```python
from build123d import *

# Parameters (mm, degrees)
F1_DEPTH = 9.525
F2_R     = 2
F3_DEPTH = 1.6002
F5_DEPTH = 1.6002
F6_R     = 2.0447
F6_R_2   = 2.05
F7_DEPTH = 1.6002


# Not quite as in the source:
# - a feature names something its author has since deleted; it is built from what else it names


with BuildPart() as f1:
    # F0 (on Front) → F1 (new body, symmetric)
    with BuildSketch(Plane.XZ):
        Polygon((1.6002, 19.05), (0, 19.05), (0, 0), (20.6502, 0), (20.6502, 1.6002), (1.6002, 1.6002), align=None)
    extrude(amount=F1_DEPTH, both=True)

    # F2 (on face) → F3 (cut, through all)
    with BuildSketch(Plane(origin=(0, 0, 0), x_dir=(0, -1, 0), z_dir=(-1, 0, 0))):
        with Locations((0, 11.43)):
            Circle(F2_R)
    extrude(amount=-F3_DEPTH, mode=Mode.SUBTRACT)

    # F4 (on face) → F5 (cut, through all)
    with BuildSketch(Plane(origin=(0, 0, 0), x_dir=(0, -1, 0), z_dir=(-1, 0, 0))):
        with BuildLine():
            Line((-9.525, 19.05), (-9.525, 1.6002))
            Line((-9.525, 1.6002), (-4.6136292969, 13.3572842838))
            ThreePointArc((-4.6136292969, 13.3572842838), (-2.7716041006, 15.5915154343), (0, 16.43))
            ThreePointArc((0, 16.43), (2.7716041006, 15.5915154343), (4.6136292969, 13.3572842838))
            Line((4.6136292969, 13.3572842838), (9.525, 1.6002))
            Line((9.525, 1.6002), (9.525, 19.05))
            Line((9.525, 19.05), (-9.525, 19.05))
        make_face()
    extrude(amount=-F5_DEPTH, mode=Mode.SUBTRACT)

    # F6 (on face) → F7 (cut, through all)
    with BuildSketch(Plane.XY.offset(1.6002)):
        with Locations((13.0302, 5.08)):
            Circle(F6_R)
        with Locations((9.2202, -4.445)):
            Circle(F6_R_2)
    extrude(amount=-F7_DEPTH, mode=Mode.SUBTRACT)


solid = f1.part
```
Check sheet for the modelled part. Datum: model origin and axes. Units: mm. A direction names the side the tool comes from. Coordinates: 2 decimals unless noted, no trailing zeros. Order: outer loops, then holes, each group sorted by start corner. A loop starts at its lowest first (then second) coordinate and runs counter-clockwise, first axis right, second up. Notation, with made-up numbers: (-35, 24) -> (-13, 24) arc R4 ccw to (-13, 30) -> close; hole circle Ø11 at (7.5, -14.5). An arc over 180 degrees is marked (long way). Write each question's results on one line, items separated by ' | '. Start each with the question number.
1) Section check C-C (x = 13). Enter the section's corners in (y, z) (3 decimals).
2) Draft check along X on faces 1 (the face through (0.789, -7.035, 7.561)), 2 (the face through (10.987, 5.17, 0.811)), 3 (the face through (0, 0, 7)). Enter one of: pulls with the +X half, pulls with the -X half, needs draft (parallel to the pull), parting line crosses it, or undercut.
3) Set-up check for faces 4 (the face through (0.789, 0.26, 13.413)), 5 (the face through (11, 0, 1.6)): record each of +Z, -Z, +X, -X, +Y, -Y from which the full face is reachable in a straight line by a thin tool's end or side.
4) Section check D-D (x = 16). Enter the section's corners in (y, z) (3 decimals).
5) Section check B-B (z = 10). Enter the section's corners in (x, y), and give its area (3 significant figures).
6) Section check A-A (y = 5.08). Enter the section's corners in (x, z).
7) Material ranges on line 1 along Z through (x, y) = (1.05, 0); line 2 along Z through (x, y) = (6.25, -7), recorded low to high.
8) Depth check by flat-ended pin: pin 1 (3 mm diameter, centred on y = 0, z = 11.43, fed in from +X); pin 2 (6 mm diameter, centred on x = 18, y = -4.5, fed in from +Z); pin 3 (8 mm diameter, centred on x = 14, y = -7, fed in from -Z); pin 4 (3 mm diameter, centred on y = 3, z = 10.5, fed in from +X). Enter the tip coordinate at first touch or a pass-through.
Checked values:
1) outline: (-9.525, 0) -> (3.036, 0) -> (3.036, 1.6) -> (-9.525, 1.6) -> close; (7.124, 0) -> (9.525, 0) -> (9.525, 1.6) -> (7.124, 1.6) -> close
2) face 1: needs draft | face 2: undercut | face 3: pulls with the -X half
3) face 4: +X, -X | face 5: +Z, +X, +Y, -Y
4) outline: (-9.525, 0) -> (9.525, 0) -> (9.525, 1.6) -> (-9.525, 1.6) -> close
5) outline: (0, -6.02) -> (1.6, -6.02) -> (1.6, -1.4) -> (0, -1.4) -> close; (0, 1.4) -> (1.6, 1.4) -> (1.6, 6.02) -> (0, 6.02) -> close | area: 14.8 mm²
6) outline: (0, 0) -> (10.99, 0) -> (10.99, 1.6) -> (1.6, 1.6) -> (1.6, 12.24) -> (0, 12.24) -> close; (15.07, 0) -> (20.65, 0) -> (20.65, 1.6) -> (15.07, 1.6) -> close
7) line 1: 0 to 9.43, 13.43 to 16.43 | line 2: 0 to 1.6
8) pin 1: through | pin 2: z = 1.6 | pin 3: z = 0 | pin 4: x = 1.6
